Autodesk Inventor part; units mm, degrees
ref_plane "YZ Plane" through (0, 0, 0) normal (1, 0, 0) x (0, 1, 0)
ref_plane "XZ Plane" through (0, 0, 0) normal (0, 1, 0) x (-1, 0, 0)
ref_plane "XY Plane" through (0, 0, 0) normal (0, 0, 1) x (1, 0, 0)
sketch "Sketch1" plane through (0, 0, 0) normal (0, 0, 1) x (1, 0, 0)
  circle A0 centre (0, 0) radius 7.4168
  circle A1 centre (0, 0) radius 10.8839
  dimension "d0" = 14.8336
  dimension "d1" = 21.7678
extrude "Extrusion1" add sketch "Sketch1" along normal blind 90.8812
sketch "Sketch2" plane through (0, 0, 90.8812) normal (0, 0, 1) x (1, 0, 0)
  circle A0 centre (0, 0) radius 10.8839
  circle A1 centre (0, 0) radius 9.662
extrude "Extrusion2" cut sketch "Sketch2" against normal blind 12.7
thread "Thread2"
sketch "Sketch4" plane through (0, 0, 0) normal (0, 0, -1) x (-1, 0, 0)
  circle A0 centre (0, 0) radius 10.8839
  circle A1 centre (0, 0) radius 9.6647
  circle A2 centre (0, 0) radius 10.8839
  dimension "d13" = 19.3294
extrude "Extrusion4" cut sketch "Sketch4" against normal blind 12.7
thread "Thread3"
properties part number "Pipe2"
Model file for the job. Use its own axes, mm. A direction names the side the tool comes from. Give positions to 0.01 mm unless a question says otherwise; leave off trailing zeros. Order: outer loops, then holes, each group sorted by start corner. A loop starts at its lowest first (then second) coordinate and runs counter-clockwise, first axis right, second up. Notation, with made-up numbers: M 30,-1 L 75,-1 A18 cw 75,18 Z; hole C 30.25,-14 d8. An arc over 180 degrees is marked long. Write item = value, one per line.
Q1. Cut at C-C, the plane z = 76.5. List the corners of the cut face in (x, y).
Derived:
outline = C 0,0 d21.77; hole C 0,0 d14.83
Q2. Cut at A-A, the plane x = 0. List the corners of the cut face in (y, z), then the cut area to 3 significant figures.
Derived:
outline = M -10.88,12.7 L -9.66,12.7 L -9.66,0 L -7.42,0 L -7.42,90.88 L -9.66,90.88 L -9.66,78.18 L -10.88,78.18 Z; M 7.42,0 L 9.66,0 L 9.66,12.7 L 10.88,12.7 L 10.88,78.18 L 9.66,78.18 L 9.66,90.88 L 7.42,90.88 Z
area = 568 mm2
Q3. Drill centre lines: line 1 (Y direction, x = -0.5, z = 41.5); line 2 (X direction, y = 3, z = 28); line 3 (Y direction, x = -4.25, z = 56). Where is each one in solid material? Low to high. Write a range as [from, to].
Derived:
line_1 = [-10.87, -7.4], [7.4, 10.87]
line_2 = [-10.46, -6.78], [6.78, 10.46]
line_3 = [-10.02, -6.08], [6.08, 10.02]
Q4. Flat gauge pins, fed straight in: pin 1 (2 mm diameter, centred on x = -1.5, z = 33, fed in from -Y); pin 2 (2 mm diameter, centred on y = 3.5, z = 23.5, fed in from -X); pin 3 (6 mm diameter, centred on x = -7.5, z = 38.5, fed in from +Y). Where does each tip first touch, or does it go through?
Derived:
pin_1 = -10.87
pin_2 = -10.59
pin_3 = 9.91
Q5. Tool access for faces 1 (the cylindrical face through (-9.22, 2.9, 6.26)), 2 (the cylindrical face through (-2.095, -9.432, 84.62)), 3 (the cylindrical face through (-2.359, 10.625, 44.982)): list every direction of +Z, -Z, +X, -X, +Y, -Y with a clear straight run to the whole face (end or side of a thin tool).
Derived:
face_1 = -Z
face_2 = +Z
face_3 = +Z, -Z
